from build123d import *

# Parameters (mm, degrees)
F0_R         = 75.6647788215
F0_R_2       = 67.1352595914
F1_DEPTH     = 25
F2_DEPTH     = 25
F1_FACE_R    = 75.6647788215
F1_FACE_R_2  = 67.1352595914
F1_FACE1_R   = 75.6647788215
F1_FACE1_R_2 = 67.1352595914
F3_R         = 75.5867204447
F3_R_2       = 67.1352595914
F4_DEPTH     = 50


with BuildPart() as f1:
    # F0 (on Top) → F1 (new body)
    with BuildSketch(Plane.XY):
        Circle(F0_R)
        Circle(F0_R_2, mode=Mode.SUBTRACT)
    extrude(amount=F1_DEPTH)

    # F0 (on Top) → F2 (join)
    with BuildSketch(Plane.XY):
        Circle(F0_R)
        Circle(F0_R_2, mode=Mode.SUBTRACT)
    extrude(amount=F2_DEPTH)

    # F1_face (on face) + F1_face1 (on face) + F3 (on face) → F4 (join)
    with BuildSketch(Plane(origin=(0, 0, 0), x_dir=(1, 0, 0), z_dir=(0, 0, -1))):
        Circle(F1_FACE_R)
        Circle(F1_FACE_R_2, mode=Mode.SUBTRACT)
    with BuildSketch(Plane.XY.offset(25)):
        Circle(F1_FACE1_R)
        Circle(F1_FACE1_R_2, mode=Mode.SUBTRACT)
    with BuildSketch(Plane(origin=(0, 0, 0), x_dir=(1, 0, 0), z_dir=(0, 0, -1))):
        Circle(F3_R)
        Circle(F3_R_2, mode=Mode.SUBTRACT)
        Circle(F3_R_2)
    extrude(amount=F4_DEPTH, dir=(0, 0, -1))


solid = f1.part
The model under review builds one solid part; all positions refer to its coordinate system, in mm. Give positions to 0.01 mm unless a question says otherwise; leave off trailing zeros. Order: outer loops, then holes, each group sorted by start corner. A loop starts at its lowest first (then second) coordinate and runs counter-clockwise, first axis right, second up. Notation, with made-up numbers: M -2.75,25 L 31.25,25 A28 cw 31.25,52 Z; hole C 57.25,-10.5 d6. An arc over 180 degrees is marked long. Answer in a Markdown table with one row per item. Add a question column.
1. Mouldability with a two-part tool opening along X and no side actions: class faces 1 (the flat face through (-1, -1, 0)), 2 (the flat face through (-1, -1, -50)), 3 (the cylindrical face through (64.035, 20.166, 12.325)), 4 (the cylindrical face through (72.17, -22.73, -11.98)) as released by +X, released by -X, zero draft, split by the parting line, or undercut.
2. To check wall thickness, follow line 1 along Y through (x, z) = (0, 7); line 2 along Z through (x, y) = (17, 44); line 3 along Y through (x, z) = (-12, 6). State the ranges of each line that lie inside material, in increasing order.
3. Add section C-C on z = -34.5. State the section outline as (x, y) points, plus the area to 3 significant figures.
4. For pin 1 Ø1.5 at (x, z) = (15.5, -0.5) entering from -Y; pin 2 Ø12 at (x, z) = (11, -29.5) entering from +Y; pin 3 Ø5 at (x, y) = (-60, 9) entering from +Z, all flat-tipped, find the tip position at first contact; note any pin that passes through.
5. Add section A-A on y = 0. State the section outline as (x, z) points, plus the area to 3 significant figures.
6. Add section D-D on z = 16. State the section outline as (x, y) points, plus the area to 3 significant figures.
The answers:
| question | item | result |
|---|---|---|
| 1 | face 1 | undercut |
| 1 | face 2 | zero draft |
| 1 | face 3 | undercut |
| 1 | face 4 | split by the parting line |
| 2 | line 1 | -75.66 to -67.14, 67.14 to 75.66 |
| 2 | line 2 | -50 to 0 |
| 2 | line 3 | -74.71 to -66.05, 66.05 to 74.71 |
| 3 | outline | C 0,0 d151.33 |
| 3 | area | 18,000 mm2 |
| 4 | pin 1 | y = -74.21 |
| 4 | pin 2 | y = 75.5 |
| 4 | pin 3 | z = 0 |
| 5 | outline | M -75.66,-50 L 75.66,-50 L 75.66,25 L 67.14,25 L 67.14,0 L -67.14,0 L -67.14,25 L -75.66,25 Z |
| 5 | area | 7,990 mm2 |
| 6 | outline | C 0,0 d151.33; hole C 0,0 d134.27 |
| 6 | area | 3,830 mm2 |
